```python
from build123d import *

# Parameters (mm, degrees)
SKETCH3_R           = 1.5
SKETCH3_R_2         = 2.5
BOSS_EXTRUDE2_DEPTH = 2.5


with BuildPart() as part:
    # Sketch3 → Boss-Extrude2 (new body)
    with BuildSketch(Plane(origin=(0, 0, 0), x_dir=(1, 0, 0), z_dir=(0, 1, 0))):
        Polygon((-68.1, 70.5), (-58.1, 70.5), (-58.1, -30), (58.1, -30), (58.1, 70.5), (68.1, 70.5), (68.1, -50), (-68.1, -50), align=None)
        with Locations(Location((-63.1, 65.5, 0), (0, 0, 270))):
            Circle(SKETCH3_R, mode=Mode.SUBTRACT)
        with Locations(Location((-63.1, 0, 0), (0, 0, 270))):
            Circle(SKETCH3_R, mode=Mode.SUBTRACT)
        with Locations(Location((63.1, 0, 0), (0, 0, 90))):
            Circle(SKETCH3_R, mode=Mode.SUBTRACT)
        with Locations(Location((63.1, 65.5, 0), (0, 0, 90))):
            Circle(SKETCH3_R, mode=Mode.SUBTRACT)
        with Locations(Location((-15, -40, 0), (0, 0, 270))):
            Circle(SKETCH3_R_2, mode=Mode.SUBTRACT)
        with Locations(Location((15, -40, 0), (0, 0, 90))):
            Circle(SKETCH3_R_2, mode=Mode.SUBTRACT)
    extrude(amount=BOSS_EXTRUDE2_DEPTH)


solid = part.part
```
Build history of the part. All positions in model axes, mm. Round coordinates to 2 decimals unless told otherwise and drop trailing zeros. Write each loop counter-clockwise with the first axis right and the second up, starting at its lowest first coordinate (ties: lowest second). Pieces come first, ordered by that corner, then holes.
1) Band-saw the part on B-B, the plane x = 63.1. List the corners of the cut face in (y, z).
2) Drill centre lines: probe 1 along X at (y, z) = (0.75, 40); probe 2 along X at (y, z) = (1.65, -65.5); probe 3 along X at (y, z) = (1.8, -54.5). Where is each one in solid material? Low to high.
3) Band-saw the part on C-C, the plane z = -20. List the corners of the cut face in (x, y), and give its area (3 significant figures).
4) Mould opens along Z. For faces 1 (the flat face through (-5, 2.5, 34)), 2 (the cylindrical face through (-61.613, 1.232, -0.195)), 3 (the cylindrical face through (61.613, 1.232, 0.195)) say: +Z half, -Z half, draft (parallel to the pull), parting line (faces both ways), or undercut.
5) Band-saw the part on A-A, the plane x = -15. List the corners of the cut face in (y, z).
6) Band-saw the part on D-D, the plane y = 1.1. List the corners of the cut face in (x, z).
Ans:
1. outline: (0, -70.5) - (2.5, -70.5) - (2.5, -67) - (0, -67) - close; (0, -64) - (2.5, -64) - (2.5, -1.5) - (0, -1.5) - close; (0, 1.5) - (2.5, 1.5) - (2.5, 50) - (0, 50) - close
2. probe 1: x = -68.1 to -17.5, -12.5 to 12.5, 17.5 to 68.1
2. probe 2: x = -68.1 to -64.6, -61.6 to -58.1, 58.1 to 61.6, 64.6 to 68.1
2. probe 3: x = -68.1 to -58.1, 58.1 to 68.1
3. outline: (-68.1, 0) - (-58.1, 0) - (-58.1, 2.5) - (-68.1, 2.5) - close; (58.1, 0) - (68.1, 0) - (68.1, 2.5) - (58.1, 2.5) - close
3. area: 50.0 mm2
4. face 1: draft
4. face 2: undercut
4. face 3: undercut
5. outline: (0, 30) - (2.5, 30) - (2.5, 37.5) - (0, 37.5) - close; (0, 42.5) - (2.5, 42.5) - (2.5, 50) - (0, 50) - close
6. outline: (-68.1, -70.5) - (-58.1, -70.5) - (-58.1, 30) - (58.1, 30) - (58.1, -70.5) - (68.1, -70.5) - (68.1, 50) - (-68.1, 50) - close; hole circle Ø3 at (-63.1, -65.5); hole circle Ø3 at (-63.1, 0); hole circle Ø5 at (-15, 40); hole circle Ø5 at (15, 40); hole circle Ø3 at (63.1, -65.5); hole circle Ø3 at (63.1, 0)
